Autodesk Inventor part; units mm, degrees
ref_plane "YZ Plane" through (0, 0, 0) normal (1, 0, 0) x (0, 1, 0)
ref_plane "XZ Plane" through (0, 0, 0) normal (0, 1, 0) x (-1, 0, 0)
ref_plane "XY Plane" through (0, 0, 0) normal (0, 0, 1) x (1, 0, 0)
sketch "Sketch1" plane through (0, 0, 0) normal (0, 1, 0) x (-1, 0, 0)
  line L0 (0, 0) -> (-28, 0)
  line L1 (-28, 0) -> (-28, -25)
  line L2 (-28, -25) -> (0, -25)
  line L3 (0, -25) -> (0, 0)
  line L4 (-24.8835, -25) -> (-24.8835, 0) construction
  line L5 (0, -1.9376) -> (-28, -1.9376) construction
  line L6 (-2.7003, -25) -> (-2.7003, 0) construction
  line L7 (0, -22.688) -> (-28, -22.688) construction
  line L8 (-34, -12.5) -> (0, -12.5) construction
  circle A0 centre (-34, -12.5) radius 6
  circle A1 centre (-34, -12.5) radius 9
  dimension "d0" = 28
  dimension "d1" = 25
  dimension "d31" = 12
  dimension "d32" = 12.5
  dimension "d33" = 18
extrude "Extrusion1" add sketch "Sketch1" along normal blind 10 contours L3 L2 L1 A1 L0 | A1 L1 picked at (-27.5773, -8.4946)
sketch "Sketch2" plane through (0, 0, 0) normal (0, 0, 1) x (1, 0, 0)
  line L0 (0, 0) -> (28, 0)
  line L1 (28, 0) -> (28, 10)
  line L2 (0, 10) -> (28, 10)
  line L3 (0, 0) -> (0, 10)
  line L4 (0, 0) -> (0, 10) construction
  line L5 (0, 2.75) -> (28, 2.75) construction
  line L6 (28, 0) -> (28, 10) construction
  circle A0 centre (14, 10.325) radius 7.575
  line L7 (0, 10) -> (28, 10) construction
  line L8 (14, 10) -> (14, 2.75) construction
  dimension "d4" = 7.25
  dimension "d5" = 15.15
extrude "Extrusion2" cut sketch "Sketch2" against normal through all contours A0 L2 | L2 A0
sketch "Sketch3" plane through (0, 10, 0) normal (0, 1, 0) x (1, 0, 0)
  line L0 (6.432, 0) -> (6.432, 25)
  line L1 (6.432, 25) -> (0, 25)
  line L2 (0, 25) -> (0, 0)
  line L3 (0, 0) -> (6.432, 0)
  line L4 (21.568, 25) -> (21.568, 0)
  line L5 (21.568, 0) -> (28, 0)
  line L6 (28, 0) -> (28, 25)
  line L7 (28, 25) -> (21.568, 25)
  line L8 (0, 21) -> (28, 21) construction
  line L9 (28, 0) -> (28, 25) construction
  line L10 (6.432, 25) -> (0, 25) construction
  line L11 (3.432, 25) -> (3.432, 0) construction
  line L12 (0, 0) -> (28, 0) construction
  line L13 (28, 25) -> (0, 25) construction
  line L14 (24.568, 25) -> (24.568, 0) construction
  line L15 (0, 25) -> (0, 0) construction
  line L16 (0, 4) -> (28, 4) construction
  circle A0 centre (3.432, 21) radius 1.625
  circle A1 centre (24.568, 21) radius 1.625
  circle A2 centre (3.432, 4) radius 1.625
  circle A3 centre (24.568, 4) radius 1.625
  dimension "d8" = 4
  dimension "d9" = 4
  dimension "d10" = 3
  dimension "d11" = 3
  dimension "d12" = 3.25
  dimension "d13" = 3.25
  dimension "d14" = 3.25
  dimension "d15" = 3.25
extrude "Extrusion3" cut sketch "Sketch3" against normal through all contours A0 | A1 | A2 | A3
chamfer "Chamfer1" distance 2.5 angle 45 4 edges at (0, 5, 0) (28, 5, 0) (28, 5, -25) (0, 5, -25)
fillet "Fillet1" radius 1 30 edges at (14, 0, -25) (2.5, 5, -25) (0, 5, -22.5) (1.25, 0, -23.75) (14, 2.75, -25) (14, 2.75, 0) (6.432, 10, -12.5) (21.568, 10, -12.5) (0, 10, -12.5) (1.25, 10, -1.25) (4.466, 10, 0) (4.466, 10, -25) (1.25, 10, -23.75) (23.534, 10, -25) (25.5, 5, -25) (28, 5, -22.5) (26.75, 0, -23.75) (26.75, 10, -23.75) (28, 10, -12.5) (26.75, 10, -1.25) (23.534, 10, 0) (28, 0, -12.5) (28, 5, -2.5) (26.75, 0, -1.25) (14, 0, 0) (1.25, 0, -1.25) (0, 0, -12.5) (25.5, 5, 0) (2.5, 5, 0) (0, 5, -2.5)
sketch "Sketch5" plane through (0, 0, 0) normal (0, -1, 0) x (1, 0, 0)
  circle A0 centre (3.432, -4) radius 1.625
  circle A1 centre (3.432, -4) radius 2.375
  circle A2 centre (3.432, -21) radius 1.625
  circle A3 centre (24.568, -21) radius 1.625
  circle A4 centre (24.568, -4) radius 1.625
  circle A5 centre (3.432, -21) radius 2.375
  circle A6 centre (24.568, -21) radius 2.375
  circle A7 centre (24.568, -4) radius 2.375
  point P0 (0, 0)
  dimension "d22" = 4.75
  dimension "d23" = 4.75
  dimension "d24" = 4.75
  dimension "d25" = 4.75
extrude "Extrusion4" cut sketch "Sketch5" against normal blind 5
equation "\"d9\" = d8"
equation "\"d11\" = d10"
equation "\"d13\" = d12"
equation "\"d14\" = d12"
equation "\"d15\" = d12"
properties part number "hotend_holder_pulley" material "ABS Plastic"
Work out the finished part from the listing and answer in its coordinate system (mm). A direction names the side the tool comes from. Give positions to 0.01 mm unless a question says otherwise; leave off trailing zeros. Write each loop counter-clockwise with the first axis right and the second up, starting at its lowest first coordinate (ties: lowest second). Pieces come first, ordered by that corner, then holes. Notation, with made-up numbers: (89, -19) - (146, -19) arc R11 ccw to (146, 0) - close; hole circle Ø6 at (-4, 79). An arc over 180 degrees is marked (long way). Use one line per item in the form item = value.
1. Consider L1, parallel to X at y = 4.5, z = -23; L2, parallel to Z at x = 26.5, y = 1.25; L3, parallel to Z at x = 23.25, y = 2.25. Determine where each line is inside the solid, lowest interval first.
Filled in:
L1 = 0.5 to 2.15, 4.71 to 9.16, 18.84 to 23.29, 25.85 to 27.5
L2 = -24 to -22.38, -19.62 to -5.38, -2.62 to -1
L3 = -25 to -22.98, -19.02 to -5.98, -2.02 to 0
2. A cutting plane is placed at C-C (z = -9.75). Write down the section's boundary in (x, y) (3 decimals), and give its area (3 significant figures).
Filled in:
outline = (0, 1) arc R1 ccw to (1, 0) - (27, 0) arc R1 ccw to (28, 1) - (28, 9) arc R1 ccw to (27, 10) - (22.472, 10) arc R1 ccw to (21.484, 9.155) arc R7.575 cw to (6.516, 9.155) arc R1 ccw to (5.528, 10) - (1, 10) arc R1 ccw to (0, 9) - close
area = 194 mm^2
3. A cutting plane is placed at B-B (y = 9.5). Write down the section's boundary in (x, z) (3 decimals), and give its area (3 significant figures).
Filled in:
outline = (0.134, -22.086) arc R0.866 ccw to (0.388, -22.698) - (2.302, -24.612) arc R0.866 ccw to (2.914, -24.866) - (5.528, -24.866) arc R0.866 ccw to (6.394, -24) - (6.394, -1) arc R0.866 ccw to (5.528, -0.134) - (2.914, -0.134) arc R0.866 ccw to (2.302, -0.388) - (0.388, -2.302) arc R0.866 ccw to (0.134, -2.914) - close; (21.606, -24) arc R0.866 ccw to (22.472, -24.866) - (25.086, -24.866) arc R0.866 ccw to (25.698, -24.612) - (27.612, -22.698) arc R0.866 ccw to (27.866, -22.086) - (27.866, -2.914) arc R0.866 ccw to (27.612, -2.302) - (25.698, -0.388) arc R0.866 ccw to (25.086, -0.134) - (22.472, -0.134) arc R0.866 ccw to (21.606, -1) - close; hole circle Ø3.25 at (3.432, -21); hole circle Ø3.25 at (3.432, -4); hole circle Ø3.25 at (24.568, -21); hole circle Ø3.25 at (24.568, -4)
area = 264 mm^2
4. For faces 5 (the face through (0.285, 0.301, -12.366)), 6 (the face through (22.82, 2.46, -19.39)), 7 (the face through (21.829, 9.766, -12.339)), determine the directions among +Z, -Z, +X, -X, +Y, -Y from which every point of the face is accessible in a straight line to the end or side of a thin tool.
Filled in:
face_5 = +Z, -Z, -X, -Y
face_6 = -Y
face_7 = +Z, -Z, +Y
5. Each of these flat-tipped pins is pushed along its axis until it touches: pin 1 Ø1.9 at (x, z) = (24.568, -21) entering from -Y; pin 2 Ø1.5 at (x, z) = (8.5, -19.5) entering from -Y; pin 3 Ø3 at (x, z) = (14.5, -11) entering from +Y; pin 4 Ø2.5 at (x, z) = (4, -4.5) entering from -Y. Where does it stop, or does it pass through?
Filled in:
pin_1 = through
pin_2 = 0
pin_3 = 3.02
pin_4 = 5
6. A cutting plane is placed at D-D (z = -4.5). Write down the section's boundary in (x, y) (3 decimals).
Filled in:
outline = (0, 1) arc R1 ccw to (1, 0) - (1.11, 0) - (1.11, 5) - (1.886, 5) - (1.886, 10) - (1, 10) arc R1 ccw to (0, 9) - close; (4.978, 5) - (5.754, 5) - (5.754, 0) - (22.246, 0) - (22.246, 5) - (23.022, 5) - (23.022, 10) - (22.472, 10) arc R1 ccw to (21.484, 9.155) arc R7.575 cw to (6.516, 9.155) arc R1 ccw to (5.528, 10) - (4.978, 10) - close; (26.114, 5) - (26.89, 5) - (26.89, 0) - (27, 0) arc R1 ccw to (28, 1) - (28, 9) arc R1 ccw to (27, 10) - (26.114, 10) - close
7. Determine the mould class of faces 1 (the face through (2.234, 7.535, -5.098)), 2 (the face through (1.3, 5.1, -1.2)), 3 (the face through (28, 5, -12)), 4 (the face through (3, 10, -12)) for opening direction X: released by +X, released by -X, zero draft, split by the parting line, or undercut.
Filled in:
face_1 = undercut
face_2 = released by -X
face_3 = released by +X
face_4 = zero draft
8. A cutting plane is placed at A-A (z = -21). Write down the section's boundary in (x, y) (3 decimals).
Filled in:
outline = (0, 1) arc R1 ccw to (1, 0) - (1.057, 0) - (1.057, 5) - (1.807, 5) - (1.807, 10) - (1, 10) arc R1 ccw to (0, 9) - close; (5.057, 5) - (5.807, 5) - (5.807, 0) - (22.193, 0) - (22.193, 5) - (22.943, 5) - (22.943, 10) - (22.472, 10) arc R1 ccw to (21.484, 9.155) arc R7.575 cw to (6.516, 9.155) arc R1 ccw to (5.528, 10) - (5.057, 10) - close; (26.193, 5) - (26.943, 5) - (26.943, 0) - (27, 0) arc R1 ccw to (28, 1) - (28, 9) arc R1 ccw to (27, 10) - (26.193, 10) - close
